Could you check a few things on this drawing? It's one solid part, dimensions in mm from its lowest x, y, z. Give positions to 0.01 mm unless a question says otherwise; leave off trailing zeros. Loops run counter-clockwise (first coordinate to the right, second up) from the corner with the lowest first, then second, coordinate; pieces in that order, holes last. Notation, with made-up numbers: (-26.5, 31) - (23.5, 31) arc R25 ccw to (23.5, 50) - close; hole circle Ø10 at (27, 57.25). An arc over 180 degrees is marked (long way). Use a Markdown table: item, result.
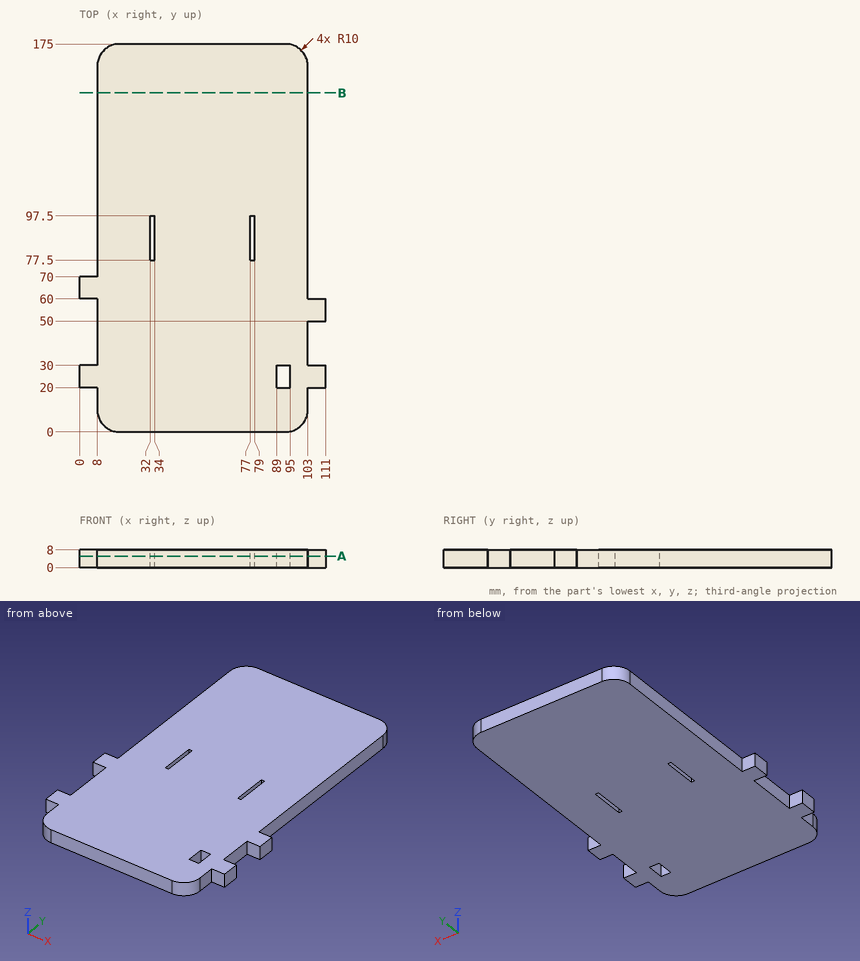
(1) Will these pins go through, and if not, where does the flat tip stop? pin 1 (2.5 mm diameter, centred on x = 105.5, z = 6, fed in from +Y); pin 2 (4 mm diameter, centred on x = 105.5, z = 5.5, fed in from -Y); pin 3 (4 mm diameter, centred on y = 104.5, z = 2, fed in from -X).
A:
| item | result |
|---|---|
| pin 1 | y = 60 |
| pin 2 | y = 20 |
| pin 3 | x = 8 |
(2) If I drill on line 1 (X direction, y = 95, z = 4); line 2 (Y direction, x = 89.5, z = 4.75); line 3 (X direction, y = 63, z = 2), over which ranges is the centre line in solid material (lowest first)?
A:
| item | result |
|---|---|
| line 1 | 8 to 32, 34 to 77, 79 to 103 |
| line 2 | 0 to 20, 30 to 175 |
| line 3 | 0 to 103 |
(3) Suppose I cut it at B-B on y = 153. Write out the boundary of the cut face in (x, z), plus the area to 3 significant figures.
A:
| item | result |
|---|---|
| outline | (8, 0) - (103, 0) - (103, 8) - (8, 8) - close |
| area | 760 mm2 |
(4) Suppose I cut it at A-A on z = 5.25. Count the separate pieces of the cut face and the enclosed holes in it, plus the area to 3 significant figures.
A:
| item | result |
|---|---|
| separate pieces | 1 |
| enclosed holes | 3 |
| area | 16,700 mm2 |
